```python
from build123d import *

# Parameters (mm, degrees)
SKETCH1_W           = 441.979400076
SKETCH1_H           = 305.81676
BOSS_EXTRUDE1_DEPTH = 2.54
CUT_EXTRUDE1_DEPTH  = 271.648139079
LPATTERN1_COUNT     = 3
LPATTERN1_PITCH     = 181.613999992
CUT_EXTRUDE2_DEPTH  = 271.648139079
LPATTERN2_COUNT     = 2
LPATTERN2_PITCH     = 181.613999992
CUT_EXTRUDE3_DEPTH  = 271.648139079


with BuildPart() as part:
    # Sketch1 → Boss-Extrude1 (new body)
    # profile 1 of 5: a face of its own
    with BuildSketch(Plane.XY):
        with Locations((0, -3.32067)):
            Rectangle(SKETCH1_W, SKETCH1_H)
        with BuildLine():
            ThreePointArc((-98.112625, -113.8), (-97.233945344, -115.921320344), (-95.112625, -116.8))
            Line((-95.112625, -116.8), (-75.712625, -116.8))
            ThreePointArc((-75.712625, -116.8), (-73.591304656, -115.921320344), (-72.712625, -113.8))
            Line((-72.712625, -113.8), (-72.712625, -81.7))
            ThreePointArc((-72.712625, -81.7), (-73.591304656, -79.578679656), (-75.712625, -78.7))
            Line((-75.712625, -78.7), (-95.112625, -78.7))
            ThreePointArc((-95.112625, -78.7), (-97.233945344, -79.578679656), (-98.112625, -81.7))
            Line((-98.112625, -81.7), (-98.112625, -113.8))
        make_face(mode=Mode.SUBTRACT)
        with BuildLine():
            ThreePointArc((-98.112625, 81.7), (-97.233945344, 79.578679656), (-95.112625, 78.7))
            Line((-95.112625, 78.7), (-75.712625, 78.7))
            ThreePointArc((-75.712625, 78.7), (-73.591304656, 79.578679656), (-72.712625, 81.7))
            Line((-72.712625, 81.7), (-72.712625, 113.8))
            ThreePointArc((-72.712625, 113.8), (-73.591304656, 115.921320344), (-75.712625, 116.8))
            Line((-75.712625, 116.8), (-95.112625, 116.8))
            ThreePointArc((-95.112625, 116.8), (-97.233945344, 115.921320344), (-98.112625, 113.8))
            Line((-98.112625, 113.8), (-98.112625, 81.7))
        make_face(mode=Mode.SUBTRACT)
        with BuildLine():
            ThreePointArc((-199.715375, -113.8), (-198.836695344, -115.921320344), (-196.715375, -116.8))
            Line((-196.715375, -116.8), (-177.315375, -116.8))
            ThreePointArc((-177.315375, -116.8), (-175.194054656, -115.921320344), (-174.315375, -113.8))
            Line((-174.315375, -113.8), (-174.315375, -81.7))
            ThreePointArc((-174.315375, -81.7), (-175.194054656, -79.578679656), (-177.315375, -78.7))
            Line((-177.315375, -78.7), (-196.715375, -78.7))
            ThreePointArc((-196.715375, -78.7), (-198.836695344, -79.578679656), (-199.715375, -81.7))
            Line((-199.715375, -81.7), (-199.715375, -113.8))
        make_face(mode=Mode.SUBTRACT)
        with BuildLine():
            ThreePointArc((-199.715375, 81.7), (-198.836695344, 79.578679656), (-196.715375, 78.7))
            Line((-196.715375, 78.7), (-177.315375, 78.7))
            ThreePointArc((-177.315375, 78.7), (-175.194054656, 79.578679656), (-174.315375, 81.7))
            Line((-174.315375, 81.7), (-174.315375, 113.8))
            ThreePointArc((-174.315375, 113.8), (-175.194054656, 115.921320344), (-177.315375, 116.8))
            Line((-177.315375, 116.8), (-196.715375, 116.8))
            ThreePointArc((-196.715375, 116.8), (-198.836695344, 115.921320344), (-199.715375, 113.8))
            Line((-199.715375, 113.8), (-199.715375, 81.7))
        make_face(mode=Mode.SUBTRACT)
    # profile 2 of 5: a face of its own
    with BuildSketch(Plane.XY):
        with BuildLine():
            Line((-199.715375, -113.8), (-199.715375, -81.7))
            ThreePointArc((-199.715375, -81.7), (-198.836695344, -79.578679656), (-196.715375, -78.7))
            Line((-196.715375, -78.7), (-177.315375, -78.7))
            ThreePointArc((-177.315375, -78.7), (-175.194054656, -79.578679656), (-174.315375, -81.7))
            Line((-174.315375, -81.7), (-174.315375, -113.8))
            ThreePointArc((-174.315375, -113.8), (-175.194054656, -115.921320344), (-177.315375, -116.8))
            Line((-177.315375, -116.8), (-196.715375, -116.8))
            ThreePointArc((-196.715375, -116.8), (-198.836695344, -115.921320344), (-199.715375, -113.8))
        make_face()
    # profile 3 of 5: a face of its own
    with BuildSketch(Plane.XY):
        with BuildLine():
            Line((-98.112625, -113.8), (-98.112625, -81.7))
            ThreePointArc((-98.112625, -81.7), (-97.233945344, -79.578679656), (-95.112625, -78.7))
            Line((-95.112625, -78.7), (-75.712625, -78.7))
            ThreePointArc((-75.712625, -78.7), (-73.591304656, -79.578679656), (-72.712625, -81.7))
            Line((-72.712625, -81.7), (-72.712625, -113.8))
            ThreePointArc((-72.712625, -113.8), (-73.591304656, -115.921320344), (-75.712625, -116.8))
            Line((-75.712625, -116.8), (-95.112625, -116.8))
            ThreePointArc((-95.112625, -116.8), (-97.233945344, -115.921320344), (-98.112625, -113.8))
        make_face()
    # profile 4 of 5: a face of its own
    with BuildSketch(Plane.XY):
        with BuildLine():
            Line((-199.715375, 113.8), (-199.715375, 81.7))
            ThreePointArc((-199.715375, 81.7), (-198.836695344, 79.578679656), (-196.715375, 78.7))
            Line((-196.715375, 78.7), (-177.315375, 78.7))
            ThreePointArc((-177.315375, 78.7), (-175.194054656, 79.578679656), (-174.315375, 81.7))
            Line((-174.315375, 81.7), (-174.315375, 113.8))
            ThreePointArc((-174.315375, 113.8), (-175.194054656, 115.921320344), (-177.315375, 116.8))
            Line((-177.315375, 116.8), (-196.715375, 116.8))
            ThreePointArc((-196.715375, 116.8), (-198.836695344, 115.921320344), (-199.715375, 113.8))
        make_face()
    # profile 5 of 5: a face of its own
    with BuildSketch(Plane.XY):
        with BuildLine():
            Line((-98.112625, 113.8), (-98.112625, 81.7))
            ThreePointArc((-98.112625, 81.7), (-97.233945344, 79.578679656), (-95.112625, 78.7))
            Line((-95.112625, 78.7), (-75.712625, 78.7))
            ThreePointArc((-75.712625, 78.7), (-73.591304656, 79.578679656), (-72.712625, 81.7))
            Line((-72.712625, 81.7), (-72.712625, 113.8))
            ThreePointArc((-72.712625, 113.8), (-73.591304656, 115.921320344), (-75.712625, 116.8))
            Line((-75.712625, 116.8), (-95.112625, 116.8))
            ThreePointArc((-95.112625, 116.8), (-97.233945344, 115.921320344), (-98.112625, 113.8))
        make_face()
    extrude(amount=BOSS_EXTRUDE1_DEPTH)

    # Sketch2 → Cut-Extrude1 (cut, through all)
    with BuildSketch(Plane.XY.offset(2.54)):
        with BuildLine():
            Line((-196.715375, 78.7), (-177.315375, 78.7))
            ThreePointArc((-177.315375, 78.7), (-175.194054656, 79.578679656), (-174.315375, 81.7))
            Line((-174.315375, 81.7), (-174.315375, 113.8))
            ThreePointArc((-174.315375, 113.8), (-175.194054656, 115.921320344), (-177.315375, 116.8))
            Line((-177.315375, 116.8), (-196.715375, 116.8))
            ThreePointArc((-196.715375, 116.8), (-198.836695344, 115.921320344), (-199.715375, 113.8))
            Line((-199.715375, 113.8), (-199.715375, 81.7))
            ThreePointArc((-199.715375, 81.7), (-198.836695344, 79.578679656), (-196.715375, 78.7))
        make_face()
        with BuildLine():
            Line((-199.715375, -81.7), (-199.715375, -113.8))
            ThreePointArc((-199.715375, -113.8), (-198.836695344, -115.921320344), (-196.715375, -116.8))
            Line((-196.715375, -116.8), (-177.315375, -116.8))
            ThreePointArc((-177.315375, -116.8), (-175.194054656, -115.921320344), (-174.315375, -113.8))
            Line((-174.315375, -113.8), (-174.315375, -81.7))
            ThreePointArc((-174.315375, -81.7), (-175.194054656, -79.578679656), (-177.315375, -78.7))
            Line((-177.315375, -78.7), (-196.715375, -78.7))
            ThreePointArc((-196.715375, -78.7), (-198.836695344, -79.578679656), (-199.715375, -81.7))
        make_face()
    cut_extrude1 = extrude(amount=-CUT_EXTRUDE1_DEPTH, mode=Mode.SUBTRACT)

    # LPattern1: Cut-Extrude1 ×3
    with Locations(*[(i * LPATTERN1_PITCH, 0, 0) for i in range(1, LPATTERN1_COUNT)]):
        add(cut_extrude1, mode=Mode.SUBTRACT)

    # Sketch3 → Cut-Extrude2 (cut, through all)
    with BuildSketch(Plane.XY.offset(2.54)):
        with BuildLine():
            Line((-72.712625, 81.7), (-72.712625, 113.8))
            ThreePointArc((-72.712625, 113.8), (-73.591304656, 115.921320344), (-75.712625, 116.8))
            Line((-75.712625, 116.8), (-95.112625, 116.8))
            ThreePointArc((-95.112625, 116.8), (-97.233945344, 115.921320344), (-98.112625, 113.8))
            Line((-98.112625, 113.8), (-98.112625, 81.7))
            ThreePointArc((-98.112625, 81.7), (-97.233945344, 79.578679656), (-95.112625, 78.7))
            Line((-95.112625, 78.7), (-75.712625, 78.7))
            ThreePointArc((-75.712625, 78.7), (-73.591304656, 79.578679656), (-72.712625, 81.7))
        make_face()
        with BuildLine():
            Line((-72.712625, -113.8), (-72.712625, -81.7))
            ThreePointArc((-72.712625, -81.7), (-73.591304656, -79.578679656), (-75.712625, -78.7))
            Line((-75.712625, -78.7), (-95.112625, -78.7))
            ThreePointArc((-95.112625, -78.7), (-97.233945344, -79.578679656), (-98.112625, -81.7))
            Line((-98.112625, -81.7), (-98.112625, -113.8))
            ThreePointArc((-98.112625, -113.8), (-97.233945344, -115.921320344), (-95.112625, -116.8))
            Line((-95.112625, -116.8), (-75.712625, -116.8))
            ThreePointArc((-75.712625, -116.8), (-73.591304656, -115.921320344), (-72.712625, -113.8))
        make_face()
    cut_extrude2 = extrude(amount=-CUT_EXTRUDE2_DEPTH, mode=Mode.SUBTRACT)

    # LPattern2: Cut-Extrude2 ×2
    with Locations(*[(i * LPATTERN2_PITCH, 0, 0) for i in range(1, LPATTERN2_COUNT)]):
        add(cut_extrude2, mode=Mode.SUBTRACT)

    # Sketch5 → Cut-Extrude3 (cut, through all)
    with BuildSketch(Plane.XY.offset(2.54)):
        with BuildLine():
            ThreePointArc((8.383999992, 139.78771), (7.802899846, 138.384810146), (6.399999992, 137.80371))
            Line((6.399999992, 137.80371), (1.399999992, 137.80371))
            ThreePointArc((1.399999992, 137.80371), (-1.439740841, 136.627450833), (-2.616000008, 133.78771))
            Line((-2.616000008, 133.78771), (-2.616000008, 128.78771))
            ThreePointArc((-2.616000008, 128.78771), (-1.439740841, 125.947969167), (1.399999992, 124.77171))
            Line((1.399999992, 124.77171), (6.399999992, 124.77171))
            ThreePointArc((6.399999992, 124.77171), (7.802899846, 124.190609854), (8.383999992, 122.78771))
            Line((8.383999992, 122.78771), (8.383999992, 87.77171))
            Line((8.383999992, 87.77171), (82.415999992, 87.77171))
            Line((82.415999992, 87.77171), (82.415999992, 122.78771))
            ThreePointArc((82.415999992, 122.78771), (82.997100138, 124.190609854), (84.399999992, 124.77171))
            Line((84.399999992, 124.77171), (89.399999992, 124.77171))
            ThreePointArc((89.399999992, 124.77171), (92.239740825, 125.947969167), (93.415999992, 128.78771))
            Line((93.415999992, 128.78771), (93.415999992, 133.78771))
            ThreePointArc((93.415999992, 133.78771), (92.239740825, 136.627450833), (89.399999992, 137.80371))
            Line((89.399999992, 137.80371), (84.399999992, 137.80371))
            ThreePointArc((84.399999992, 137.80371), (82.997100138, 138.384810146), (82.415999992, 139.78771))
            Line((82.415999992, 139.78771), (82.415999992, 149.80371))
            Line((82.415999992, 149.80371), (8.383999992, 149.80371))
            Line((8.383999992, 149.80371), (8.383999992, 139.78771))
        make_face()
    extrude(amount=-CUT_EXTRUDE3_DEPTH, mode=Mode.SUBTRACT)


solid = part.part
```
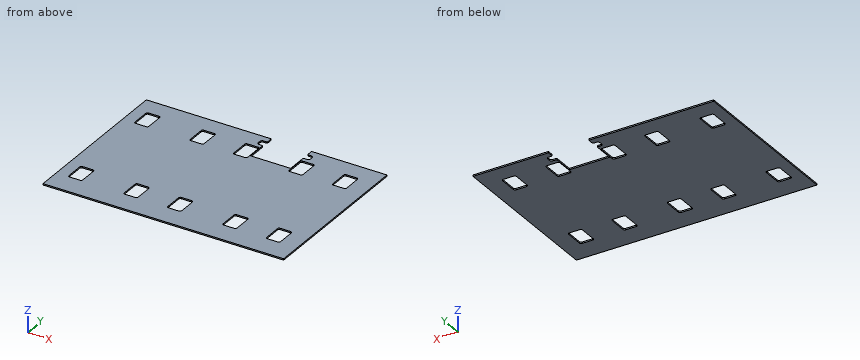
The model under review builds one solid part; all positions refer to its coordinate system, in mm. Give positions to 0.01 mm unless a question says otherwise; leave off trailing zeros. Write each loop counter-clockwise with the first axis right and the second up, starting at its lowest first coordinate (ties: lowest second). Pieces come first, ordered by that corner, then holes.
(1) Consider section B-B, the plane x = 71. Give the boundary of the cut face in (y, z).
(2) Consider section A-A, the plane z = 0.85. Give the number of separate pieces and of enclosed holes in the cut face, and give its area (3 significant figures).
(3) To check wall thickness, follow L1, parallel to Y at x = 87.5, z = 1; L2, parallel to Y at x = 168, z = 2.05; L3, parallel to X at y = -96, z = 0.75. State the ranges of each line that lie inside material, in increasing order.
Returned:
1. outline: (-156.23, 0) - (87.77, 0) - (87.77, 2.54) - (-156.23, 2.54) - close
2. separate pieces: 1
2. enclosed holes: 10
2. area: 121,000 mm2
3. L1: y = -156.23 to -116.8, -78.7 to 78.7, 116.8 to 124.77, 137.8 to 149.59
3. L2: y = -156.23 to -116.8, -78.7 to 78.7, 116.8 to 149.59
3. L3: x = -220.99 to -199.72, -174.32 to -98.11, -72.71 to -18.1, 7.3 to 83.5, 108.9 to 163.51, 188.91 to 220.99
